from build123d import *

# Parameters (mm, degrees)
SZKIC1_R                                    = 4
DODANIE_WYCI_GNI_CIE1_DEPTH                 = 119
WYTNIJ_WYCI_GNI_CIE1_REACH                  = 121.134
WYTNIJ_WYCI_GNI_CIE1_END_RADIUS             = 4
SZKIC2_R                                    = 1.5
WYTNIJ_WYCI_GNI_CIE1_DIRECTION_2_REACH      = 121.134
WYTNIJ_WYCI_GNI_CIE1_DIRECTION_2_END_RADIUS = 4
SZKIC3_R                                    = 1
DODANIE_WYCI_GNI_CIE2_DEPTH                 = 15
SZKIC4_R                                    = 2
DODANIE_WYCI_GNI_CIE3_DEPTH                 = 4
ZAOKR_GLENIE1_R                             = 2


with BuildPart() as part:
    # Szkic1 → Dodanie-wyciągnięcie1 (new body)
    with BuildSketch(Plane.XY):
        Circle(SZKIC1_R)
    extrude(amount=DODANIE_WYCI_GNI_CIE1_DEPTH)

    # Wytnij-wyciągnięcie1: up to this cylinder (the profile starts inside it)
    wytnij_wyci_gni_cie1_end = Plane(origin=(0, 0, 19.63585), z_dir=(0, 0, -1)) * Cylinder(WYTNIJ_WYCI_GNI_CIE1_END_RADIUS, 251.268, mode=Mode.PRIVATE)
    # Szkic2 → Wytnij-wyciągnięcie1 (cut, up to the surface)
    with BuildSketch(Plane(origin=(0, 0, 0), x_dir=(0, 0, -1), z_dir=(1, 0, 0)), mode=Mode.PRIVATE) as wytnij_wyci_gni_cie1_sk1:
        with Locations((-19.635850317, 0)):
            Circle(SZKIC2_R)
    wytnij_wyci_gni_cie1_tool1 = extrude(wytnij_wyci_gni_cie1_sk1.sketch, amount=-WYTNIJ_WYCI_GNI_CIE1_REACH, mode=Mode.PRIVATE) & wytnij_wyci_gni_cie1_end
    add(wytnij_wyci_gni_cie1_tool1.solids().sort_by_distance((0, 0, 19.63585))[0], mode=Mode.SUBTRACT)

    # Wytnij-wyciągnięcie1 direction 2: up to this cylinder (the profile starts inside it)
    wytnij_wyci_gni_cie1_direction_2_end = Plane(origin=(0, 0, 19.63585), z_dir=(0, 0, -1)) * Cylinder(WYTNIJ_WYCI_GNI_CIE1_DIRECTION_2_END_RADIUS, 251.268, mode=Mode.PRIVATE)
    # Szkic2 → Wytnij-wyciągnięcie1 direction 2 (cut, up to the surface)
    with BuildSketch(Plane(origin=(0, 0, 0), x_dir=(0, 0, -1), z_dir=(1, 0, 0)), mode=Mode.PRIVATE) as wytnij_wyci_gni_cie1_direction_2_sk1:
        with Locations((-19.635850317, 0)):
            Circle(SZKIC2_R)
    wytnij_wyci_gni_cie1_direction_2_tool1 = extrude(wytnij_wyci_gni_cie1_direction_2_sk1.sketch, amount=WYTNIJ_WYCI_GNI_CIE1_DIRECTION_2_REACH, mode=Mode.PRIVATE) & wytnij_wyci_gni_cie1_direction_2_end
    add(wytnij_wyci_gni_cie1_direction_2_tool1.solids().sort_by_distance((0, 0, 19.63585))[0], mode=Mode.SUBTRACT)

    # Szkic3 → Dodanie-wyciągnięcie2 (add)
    with BuildSketch(Plane.XY.offset(119)):
        Circle(SZKIC3_R)
    extrude(amount=DODANIE_WYCI_GNI_CIE2_DEPTH)

    # Szkic4 → Dodanie-wyciągnięcie3 (add)
    with BuildSketch(Plane.XY.offset(134)):
        Circle(SZKIC4_R)
    extrude(amount=DODANIE_WYCI_GNI_CIE3_DEPTH)

    # Zaokrąglenie1
    zaokr_glenie1_edges = [part.edges().sort_by_distance(p)[0] for p in [
        (-2, 0, 138),
    ]]
    fillet(zaokr_glenie1_edges, radius=ZAOKR_GLENIE1_R)


solid = part.part
Geometry: final body of the model. Coordinates: model frame, mm. A direction names the side the tool comes from. Give positions to 0.01 mm unless a question says otherwise; leave off trailing zeros. Loops run counter-clockwise (first coordinate to the right, second up) from the corner with the lowest first, then second, coordinate; pieces in that order, holes last. Notation, with made-up numbers: (19, 35) -> (58, 35) arc R22 ccw to (58, 53) -> close; hole circle Ø7 at (66.5, 88.5). An arc over 180 degrees is marked (long way). Put each result on its own line as item: value.
1. Cut plane A-A (z = 107.5). Return the cut outline in (x, y), plus the area to 3 significant figures.
Taken from the geometry:
outline: circle Ø8 at (0, 0)
area: 50.3 mm2
2. Pull-direction query (Y, two-part tool) for faces 4 (the flat face through (1, -1, 119)), 5 (the cylindrical face through (-0.056, 0.451, 18.205)), 6 (the cylindrical face through (-0.867, -3.905, 58.667)); classes: released by +Y, released by -Y, zero draft, split by the parting line, or undercut.
Taken from the geometry:
face 4: zero draft
face 5: undercut
face 6: split by the parting line
3. Set-up query: faces 1 (the flat face through (1, -1, 134)), 2 (the cylindrical face through (0, -2, 135)), 3 (the flat face through (0, 0, 0)). Return all of +Z, -Z, +X, -X, +Y, -Y with unobstructed straight access to the full face (end or side cutting, diameter ignored); none if empty.
Taken from the geometry:
face 1: none
face 2: +Z
face 3: -Z, +X, -X, +Y, -Y
4. Pin query (flat end, axial travel): P1, Ø2.5, axis at y = 0, z = 19.64, coming from the +X side. Return the tip coordinate at first contact, or that it passes through.
Taken from the geometry:
P1: passes through
5. Ray query, line 1 along Z through (x, y) = (1.75, 0); line 2 along Z through (x, y) = (-0.25, 0); line 3 along Z through (x, y) = (-1.75, 0.5). Return the intervals inside material, ascending. Write a range as [from, to].
Taken from the geometry:
line 1: z = [0, 18.14], [21.14, 119], [134, 136.97]
line 2: z = [0, 18.14], [21.14, 137.98]
line 3: z = [0, 18.22], [21.05, 119], [134, 136.83]
